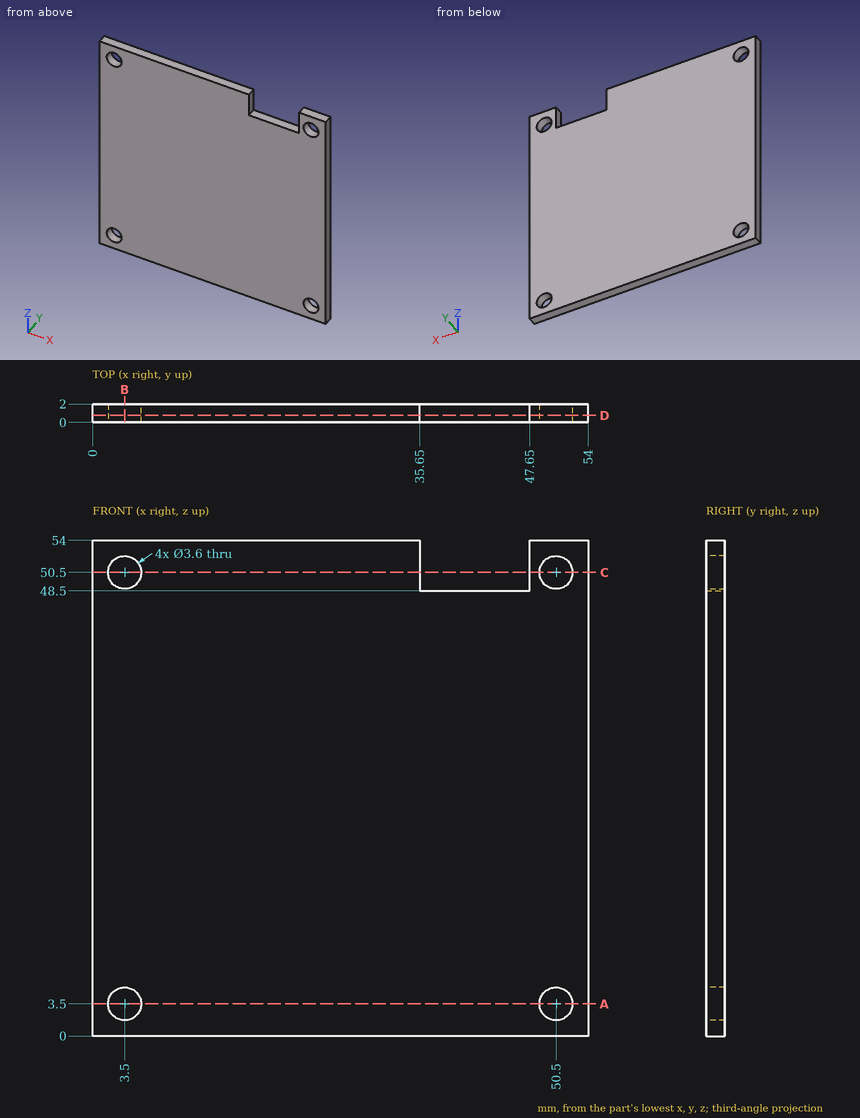
Verification items for this drawing (mm, ordinates from the low corner). Coordinates: 2 decimals unless noted, no trailing zeros. Write each loop counter-clockwise with the first axis right and the second up, starting at its lowest first coordinate (ties: lowest second). Pieces come first, ordered by that corner, then holes. Notation, with made-up numbers: M 41.5,53 L 92.5,53 A32 ccw 92.5,87 Z; hole C 44,-40 d7. An arc over 180 degrees is marked long. Answer as a JSON object with one key per item and string values. Group by question number.
(1) Cross-section at A-A, the plane z = 3.5. Record the cut outline in (x, y).
(2) Cross-section at B-B, the plane x = 3.5. Record the cut outline in (y, z).
(3) Cross-section at C-C, the plane z = 50.5. Record the cut outline in (x, y).
(4) Material ranges on line 1 (Z direction, x = 50.5, y = 0.9); line 2 (X direction, y = 0.5, z = 50.5), recorded low to high.
(5) Cross-section at D-D, the plane y = 0.75. Record the cut outline in (x, z), and give its area (3 significant figures).
Reply:
{
 "1": {"outline": "M 0,0 L 1.7,0 L 1.7,2 L 0,2 Z; M 5.3,0 L 48.7,0 L 48.7,2 L 5.3,2 Z; M 52.3,0 L 54,0 L 54,2 L 52.3,2 Z"},
 "2": {"outline": "M 0,0 L 2,0 L 2,1.7 L 0,1.7 Z; M 0,5.3 L 2,5.3 L 2,48.7 L 0,48.7 Z; M 0,52.3 L 2,52.3 L 2,54 L 0,54 Z"},
 "3": {"outline": "M 0,0 L 1.7,0 L 1.7,2 L 0,2 Z; M 5.3,0 L 35.65,0 L 35.65,2 L 5.3,2 Z; M 47.65,0 L 48.7,0 L 48.7,2 L 47.65,2 Z; M 52.3,0 L 54,0 L 54,2 L 52.3,2 Z"},
 "4": {"line 1": "0 to 1.7, 5.3 to 48.7, 52.3 to 54", "line 2": "0 to 1.7, 5.3 to 35.65, 47.65 to 48.7, 52.3 to 54"},
 "5": {"outline": "M 0,0 L 54,0 L 54,54 L 47.65,54 L 47.65,48.5 L 35.65,48.5 L 35.65,54 L 0,54 Z; hole C 3.5,3.5 d3.6; hole C 3.5,50.5 d3.6; hole C 50.5,3.5 d3.6; hole C 50.5,50.5 d3.6", "area": "2,810 mm²"}
}
